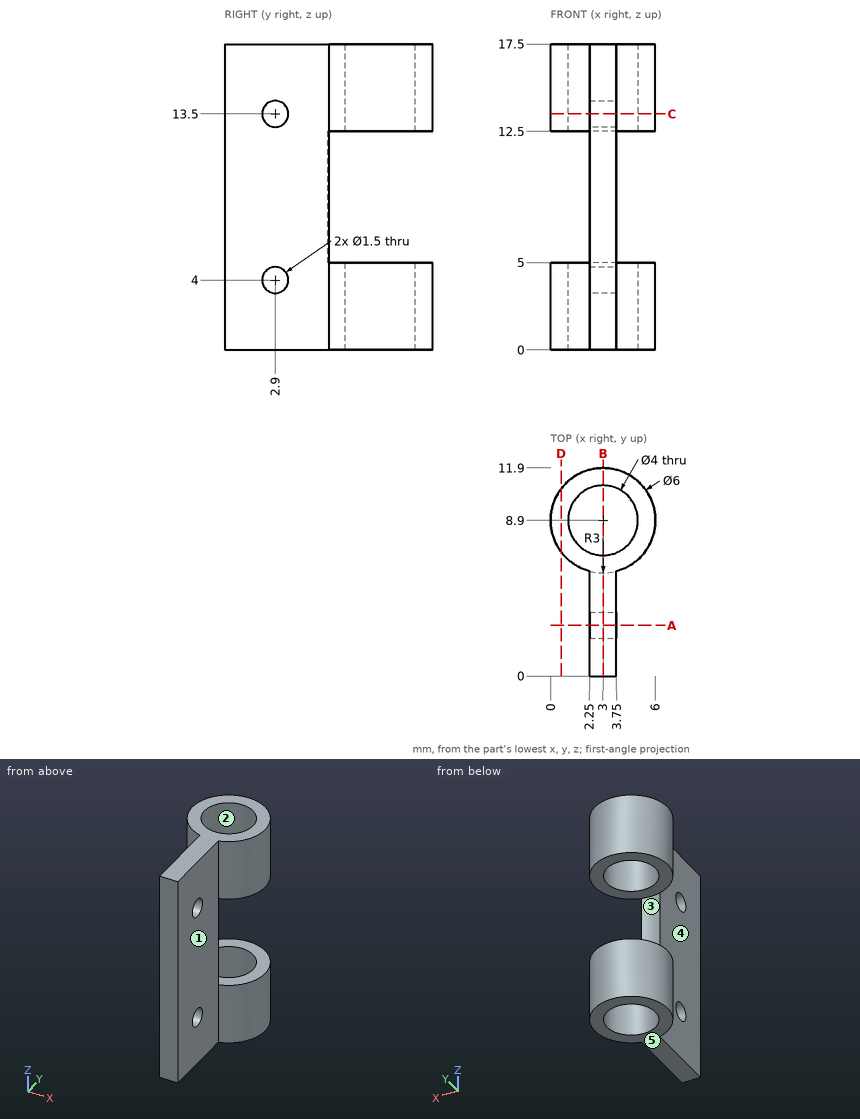
Design review of the part shown in the three views and the two pictorial views. Dimensions are in mm from the part's minimum x, y and z. A direction names the side the tool comes from. Round coordinates to 2 decimals unless told otherwise and drop trailing zeros. Write each loop counter-clockwise with the first axis right and the second up, starting at its lowest first coordinate (ties: lowest second). Pieces come first, ordered by that corner, then holes. Notation, with made-up numbers: M 0.5,33.25 L 7.5,33.25 A24 ccw 7.5,52.25 Z; hole C 45,73.25 d6. An arc over 180 degrees is marked long. Use a Markdown table: item, result. Add a question column.
Q1. We need section D-D, the plane x = 0.6. State the section outline as (y, z) points, plus the area to 3 significant figures.
Q2. We need section C-C, the plane z = 13.5. State the section outline as (x, y) points.
Q3. Insertion check: pin 1 (1.5 mm diameter, centred on y = 5.5, z = 4.5, fed in from -X); pin 2 (3 mm diameter, centred on y = 2, z = 9.5, fed in from +X); pin 3 (5 mm diameter, centred on y = 2, z = 10.5, fed in from -X). Each pin has a flat end and moves straight along its axis. Give the tip position at first contact, or say it passes through.
Q4. The part is to be moulded in two halves that separate along Z. For the marked faces 3, 4 and 5, say which applies: pulls with the +Z half, pulls with the -Z half, needs draft (parallel to the pull), parting line crosses it, or undercut.
Q5. We need section A-A, the plane y = 2.9. State the section outline as (x, z) points.
Q6. Machinability: for the marked faces 1 and 2, which of the approach directions +Z, -Z, +X, -X, +Y, -Y give a long, thin tool a straight path to every point of the face, cutting with its end or side? Answer none if there is none.
Q7. To check wall thickness, follow line 1 (Y direction, x = 3, z = 16); line 2 (Y direction, x = 3, z = 4); line 3 (Y direction, x = 3, z = 3.4). State the ranges of each line that lie inside material, in increasing order.
Q8. We need section B-B, the plane x = 3. State the section outline as (y, z) points.
Findings below:
| question | item | result |
|---|---|---|
| 1 | outline | M 7.1,0 L 10.7,0 L 10.7,5 L 7.1,5 Z; M 7.1,12.5 L 10.7,12.5 L 10.7,17.5 L 7.1,17.5 Z |
| 1 | area | 36.0 mm² |
| 2 | outline | M 2.25,0 L 3.75,0 L 3.75,2.15 L 2.25,2.15 Z; M 2.25,3.65 L 3.75,3.65 L 3.75,6 A3 ccw long 2.25,6 Z; hole C 3,8.9 d4 |
| 3 | pin 1 | stops at x = 1.59 |
| 3 | pin 2 | stops at x = 3.75 |
| 3 | pin 3 | stops at x = 2.25 |
| 4 | face 3 | undercut |
| 4 | face 4 | needs draft |
| 4 | face 5 | pulls with the -Z half |
| 5 | outline | M 2.25,0 L 3.75,0 L 3.75,3.25 L 2.25,3.25 Z; M 2.25,4.75 L 3.75,4.75 L 3.75,12.75 L 2.25,12.75 Z; M 2.25,14.25 L 3.75,14.25 L 3.75,17.5 L 2.25,17.5 Z |
| 6 | face 1 | +Z, -Z, +X, -Y |
| 6 | face 2 | +Z, -Z |
| 7 | line 1 | y = 0 to 6.9, 10.9 to 11.9 |
| 7 | line 2 | y = 0 to 2.15, 3.65 to 6.9, 10.9 to 11.9 |
| 7 | line 3 | y = 0 to 2.45, 3.35 to 6.9, 10.9 to 11.9 |
| 8 | outline | M 0,0 L 6.9,0 L 6.9,5 L 5.9,5 L 5.9,12.5 L 6.9,12.5 L 6.9,17.5 L 0,17.5 Z; M 10.9,0 L 11.9,0 L 11.9,5 L 10.9,5 Z; M 10.9,12.5 L 11.9,12.5 L 11.9,17.5 L 10.9,17.5 Z; hole C 2.9,4 d1.5; hole C 2.9,13.5 d1.5 |
